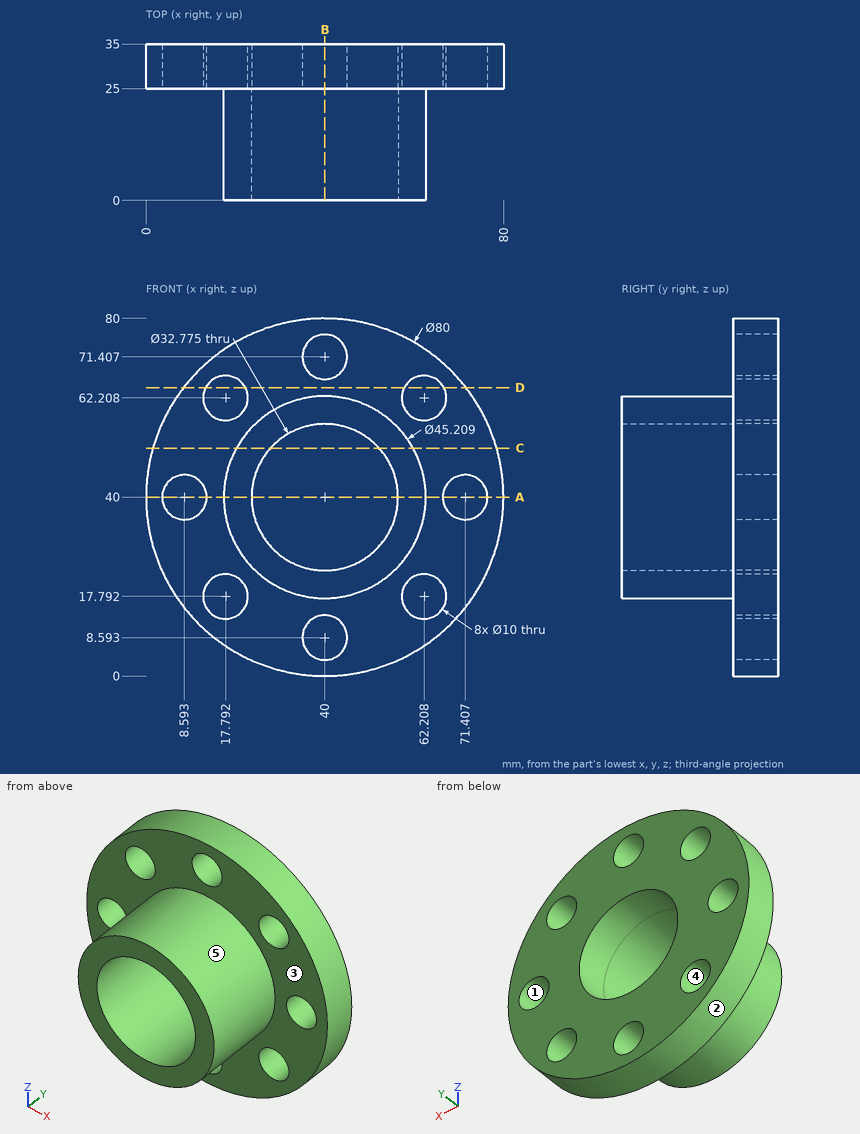
Design review of the part shown in the three views and the two pictorial views. Dimensions are in mm from the part's minimum x, y and z. A direction names the side the tool comes from. Round coordinates to 2 decimals unless told otherwise and drop trailing zeros. Write each loop counter-clockwise with the first axis right and the second up, starting at its lowest first coordinate (ties: lowest second). Pieces come first, ordered by that corner, then holes. Notation, with made-up numbers: (76.25, 76) -> (111.25, 76) arc R11 ccw to (111.25, 85) -> close; hole circle Ø6 at (80.25, -34.75). An arc over 180 degrees is marked (long way). Write item = value, one per line. Start each with the question number.
1) Tool access review of the marked faces 4 and 5: name each direction out of +Z, -Z, +X, -X, +Y, -Y from which nothing blocks a thin tool from reaching the whole face with its end or side.
2) Take a section at A-A, the plane z = 40. State the section outline as (x, y) points (1 decimal).
3) Take a section at D-D, the plane z = 64.5. State the section outline as (x, y) points, plus the area to 3 significant figures.
4) Take a section at C-C, the plane z = 51. State the section outline as (x, y) points, plus the area to 3 significant figures.
5) Clearance check with flat-ended pins moving along their axes: pin 1 (16 mm diameter, centred on x = 8.59, z = 40, fed in from +Y); pin 2 (13 mm diameter, centred on x = 17.79, z = 17.79, fed in from -Y); pin 3 (5 mm diameter, centred on x = 24, y = 15, fed in from +Z); pin 4 (1 mm diameter, centred on y = 28, z = 58, fed in from +X). State where each tip first meets the part, or that it passes through.
6) Mouldability with a two-part tool opening along X and no side actions: class the marked faces 1, 2 and 3 as +X half, -X half, draft (parallel to the pull), parting line (faces both ways), or undercut.
7) Take a section at B-B, the plane x = 40. State the section outline as (y, z) points (1 decimal), plus the area to 3 significant figures.
8) Wall thickness on probe 1 along Z at (x, y) = (40, 30); probe 2 along X at (y, z) = (33, 22) (1 decimal); probe 3 along Y at (x, z) = (61, 30.5): over which ranges is each line inside the solid? List them lowest first. Write a range as from..to.
Results list:
q1.face_4 = +Y, -Y
q1.face_5 = -Y
q2.outline = (0, 25) -> (3.6, 25) -> (3.6, 35) -> (0, 35) -> close; (13.6, 25) -> (17.4, 25) -> (17.4, 0) -> (23.6, 0) -> (23.6, 35) -> (13.6, 35) -> close; (56.4, 0) -> (62.6, 0) -> (62.6, 25) -> (66.4, 25) -> (66.4, 35) -> (56.4, 35) -> close; (76.4, 25) -> (80, 25) -> (80, 35) -> (76.4, 35) -> close
q3.outline = (8.38, 25) -> (13.35, 25) -> (13.35, 35) -> (8.38, 35) -> close; (22.24, 25) -> (57.76, 25) -> (57.76, 35) -> (22.24, 35) -> close; (66.65, 25) -> (71.62, 25) -> (71.62, 35) -> (66.65, 35) -> close
q3.area = 455 mm²
q4.outline = (1.54, 25) -> (20.25, 25) -> (20.25, 0) -> (27.85, 0) -> (27.85, 35) -> (1.54, 35) -> close; (52.15, 0) -> (59.75, 0) -> (59.75, 25) -> (78.46, 25) -> (78.46, 35) -> (52.15, 35) -> close
q4.area = 906 mm²
q5.pin_1 = 35
q5.pin_2 = 25
q5.pin_3 = 58.13
q5.pin_4 = 75.97
q6.face_1 = undercut
q6.face_2 = parting line
q6.face_3 = draft
q7.outline = (0, 17.4) -> (25, 17.4) -> (25, 13.6) -> (35, 13.6) -> (35, 23.6) -> (0, 23.6) -> close; (0, 56.4) -> (35, 56.4) -> (35, 66.4) -> (25, 66.4) -> (25, 62.6) -> (0, 62.6) -> close; (25, 0) -> (35, 0) -> (35, 3.6) -> (25, 3.6) -> close; (25, 76.4) -> (35, 76.4) -> (35, 80) -> (25, 80) -> close
q7.area = 583 mm²
q8.probe_1 = 0..3.59, 13.59..23.61, 56.39..66.41, 76.41..80
q8.probe_2 = 4.3..15.1, 20.5..59.5, 64.9..75.7
q8.probe_3 = 25..35
